Geometry check sheet. Reference: the model listing, model coordinates, mm. Face numbers are marked on the shaded views. A direction names the side the tool comes from. Give positions to 0.01 mm unless a question says otherwise; leave off trailing zeros. Order: outer loops, then holes, each group sorted by start corner. A loop starts at its lowest first (then second) coordinate and runs counter-clockwise, first axis right, second up.
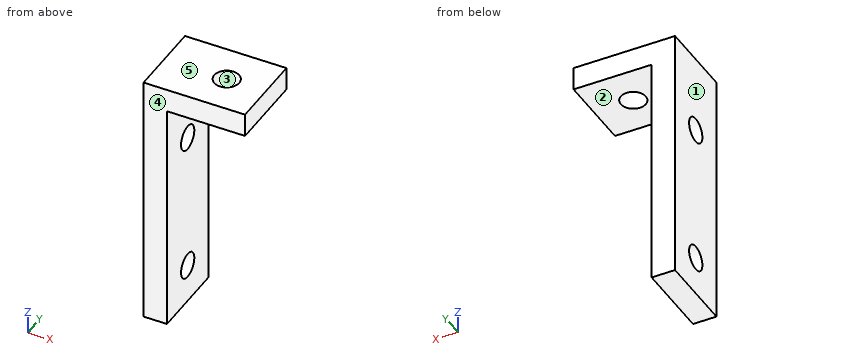
```python
from build123d import *

# Parameters (mm, degrees)
F1_DEPTH = 12.7
F3_D     = 4.064
F5_D     = 4.064


with BuildPart() as f1:
    # F0 (on Front) → F1 (new body)
    with BuildSketch(Plane.XZ):
        Polygon((0, 41.91), (0, 0), (3.81, 0), (3.81, 38.1), (16.51, 38.1), (16.51, 41.91), align=None)
    extrude(amount=F1_DEPTH)

    # F3 (through all)
    with Locations(Plane(origin=(0, 0, 38.1), x_dir=(1, 0, 0), z_dir=(0, 0, -1))):
        with Locations((10.16, 6.35)):
            Hole(F3_D / 2)

    # F5 (through all)
    with Locations(Plane.YZ.offset(3.81)):
        with Locations((-6.35, 29.21), (-6.35, 6.35)):
            Hole(F5_D / 2)


solid = f1.part
```
Q1. Thickness scan on L1, parallel to Z at x = 3, y = -6.5; L2, parallel to Z at x = 8.75, y = -8.5; L3, parallel to X at y = -7.5, z = 24. Record the ranges inside material, lowest first.
Q2. Cross-section at A-A, the plane x = 10.16. Record the boundary of the cut face in (y, z), and give its area (3 significant figures).
Q3. Cross-section at B-B, the plane y = -6.35. Record the boundary of the cut face in (x, z), and give its area (3 significant figures).
Q4. Access from +Z, -Z, +X, -X, +Y, -Y to the whole of each face (thin tool, end or side, straight path). Record for the marked faces 1 and 2.
Q5. Gauge pin test, flat ends, axial feed: P1, Ø3.5, axis at y = -6.35, z = 29.21, coming from the +X side; P2, Ø6.5, axis at x = 12.5, y = -4, coming from the -Z side. Record the tip position at first contact, or that the pin passes through.
Q6. Release check for a two-part mould opening along Y. For the marked faces 3, 4 and 5 record: pulls with the +Y half, pulls with the -Y half, needs draft (parallel to the pull), parting line crosses it, or undercut.
Q7. Cross-section at D-D, the plane y = -3.75. Record the boundary of the cut face in (x, z), and give its area (3 significant figures).
Q8. Cross-section at C-C, the plane x = 3. Record the boundary of the cut face in (y, z), and give its area (3 significant figures).
Answers follow:
1. L1: z = 0 to 4.32, 8.38 to 27.18, 31.24 to 41.91
1. L2: z = 38.1 to 41.91
1. L3: x = 0 to 3.81
2. outline: (-12.7, 38.1) - (-8.38, 38.1) - (-8.38, 41.91) - (-12.7, 41.91) - close; (-4.32, 38.1) - (0, 38.1) - (0, 41.91) - (-4.32, 41.91) - close
2. area: 32.9 mm2
3. outline: (0, 0) - (3.81, 0) - (3.81, 4.32) - (0, 4.32) - close; (0, 8.38) - (3.81, 8.38) - (3.81, 27.18) - (0, 27.18) - close; (0, 31.24) - (3.81, 31.24) - (3.81, 38.1) - (8.13, 38.1) - (8.13, 41.91) - (0, 41.91) - close; (12.19, 38.1) - (16.51, 38.1) - (16.51, 41.91) - (12.19, 41.91) - close
3. area: 162 mm2
4. face 1: +Z, -Z, -X, +Y, -Y
4. face 2: -Z, +X, +Y, -Y
5. P1: passes through
5. P2: stops at z = 38.1
6. face 3: undercut
6. face 4: pulls with the -Y half
6. face 5: needs draft
7. outline: (0, 0) - (3.81, 0) - (3.81, 38.1) - (16.51, 38.1) - (16.51, 41.91) - (0, 41.91) - close
7. area: 208 mm2
8. outline: (-12.7, 0) - (0, 0) - (0, 41.91) - (-12.7, 41.91) - close; hole circle Ø4.06 at (-6.35, 6.35); hole circle Ø4.06 at (-6.35, 29.21)
8. area: 506 mm2
